Verification items for the finished model (mm, model axes). A direction names the side the tool comes from. Give positions to 0.01 mm unless a question says otherwise; leave off trailing zeros. Order: outer loops, then holes, each group sorted by start corner. A loop starts at its lowest first (then second) coordinate and runs counter-clockwise, first axis right, second up. Notation, with made-up numbers: (88, 51) -> (114, 51) arc R30 ccw to (114, 88) -> close; hole circle Ø3 at (76, 85). An arc over 180 degrees is marked (long way). One line per question, with ' | ' between items. Start each with the question number.
Q1. Section check B-B on y = -65. Record the cut outline in (x, z), plus the area to 3 significant figures.
Q2. Material ranges on probe 1 along X at (y, z) = (-66, 213.5); probe 2 along X at (y, z) = (-25.5, 204); probe 3 along Y at (x, z) = (89.5, 183), recorded low to high. Write a range as [from, to].
Q3. Mould release check, pull along Z, two halves, no side actions. Record for faces 1 (the flat face through (17, -127, 47)), 2 (the flat face through (159, -50, -71.583)), 3 (the cylindrical face through (24.996, -50.089, 186.226)): released by +Z, released by -Z, zero draft, split by the parting line, or undercut.
Q4. Section check C-C on x = 210.5. Record the cut outline in (y, z).
Q5. Section check A-A on z = 3. Record the cut outline in (x, y).
Q6. Go/stop test with a flat-tipped pin: pin 1 (2 mm diameter, centred on x = 72.5, z = 30.5, fed in from +Y). Record where the tip stops, or that it passes through.
Q7. Access from +Z, -Z, +X, -X, +Y, -Y to the whole of each face (thin tool, end or side, straight path). Record for faces 4 (the flat face through (230, -101.6, 85)), 5 (the flat face through (159, -50, 245.917)).
from build123d import *

# Parameters (mm, degrees)
F0_W        = 139.7
F0_H        = 317.5
F0_R        = 13.2493993782
F0_R_2      = 30.8467265461
F1_DEPTH    = 127
F2_T1_DEPTH = 266.7
F2_T3_DEPTH = 444.5
F3_DEPTH    = 288.29


# Not quite as in the source:
# - a fillet or chamfer that OpenCascade refuses, or shapes differently, is made with other operations: its cross-section is extruded or revolved along the edge and cut away or added


with BuildPart() as f1:
    # F0 (on Front) → F1 (new body)
    with BuildSketch(Plane.XZ):
        with Locations((18.042704469, 87.1669226885)):
            Rectangle(F0_W, F0_H)
        with Locations((-34.4466865063, 214.674949646)):
            Circle(F0_R, mode=Mode.SUBTRACT)
        with Locations((49.4750849903, 204.995855689)):
            Circle(F0_R_2, mode=Mode.SUBTRACT)
    extrude(amount=F1_DEPTH)

    # F2: fillet of radius 25.4 on 6 edges, made by hand

    # F2_s2 → F2_t1 (cut)
    with BuildSketch(Plane.YZ.offset(-115.307295531)):
        with BuildLine():
            ThreePointArc((-101.6, 245.9169226885), (-119.5605122421, 238.4774349306), (-127, 220.5169226885))
            Line((-127, 220.5169226885), (-127, 245.9169226885))
            Line((-127, 245.9169226885), (-101.6, 245.9169226885))
        make_face()
        with BuildLine():
            ThreePointArc((-101.6, -71.5830773115), (-119.5605122421, -64.1435895537), (-127, -46.1830773115))
            Line((-127, -46.1830773115), (-127, -71.5830773115))
            Line((-127, -71.5830773115), (-101.6, -71.5830773115))
        make_face()
    extrude(amount=F2_T1_DEPTH, mode=Mode.SUBTRACT)

    # F2_s4 → F2_t3 (cut)
    with BuildSketch(Plane.XY.offset(-135.0830773115)):
        with BuildLine():
            ThreePointArc((-51.807295531, -101.6), (-44.3678077732, -119.5605122421), (-26.407295531, -127))
            Line((-26.407295531, -127), (-51.807295531, -127))
            Line((-51.807295531, -127), (-51.807295531, -101.6))
        make_face()
        with BuildLine():
            ThreePointArc((87.892704469, -101.6), (80.4532167111, -119.5605122421), (62.492704469, -127))
            Line((62.492704469, -127), (87.892704469, -127))
            Line((87.892704469, -127), (87.892704469, -101.6))
        make_face()
    extrude(amount=F2_T3_DEPTH, mode=Mode.SUBTRACT)

    # F2_s5 → F2_t6 (revolve, cut)
    with BuildSketch(Plane.XY.offset(214.674949646)):
        with BuildLine():
            ThreePointArc((-21.197287128, -101.6), (-13.7577993702, -119.5605122421), (4.202712872, -127))
            Line((4.202712872, -127), (-21.197287128, -127))
            Line((-21.197287128, -127), (-21.197287128, -101.6))
        make_face()
    revolve(axis=Axis((-34.4466865063, -127, 214.674949646), (0, -1, 0)), mode=Mode.SUBTRACT)

    # F2_s7 → F2_t8 (revolve, cut)
    with BuildSketch(Plane.XY.offset(204.995855689)):
        with BuildLine():
            ThreePointArc((80.3218115364, -101.6), (87.7612992942, -119.5605122421), (105.7218115364, -127))
            Line((105.7218115364, -127), (80.3218115364, -127))
            Line((80.3218115364, -127), (80.3218115364, -101.6))
        make_face()
    revolve(axis=Axis((49.4750849903, -127, 204.995855689), (0, -1, 0)), mode=Mode.SUBTRACT)

    # F3 (add): a face of the model
    f3_faces = [f1.faces().sort_by_distance(p)[0] for p in [
        (87.892704469, -50.8, 87.1669226885),
    ]]
    extrude(f3_faces, amount=F3_DEPTH)


solid = f1.part
Filled in:
1) outline: (-51.81, -71.58) -> (376.18, -71.58) -> (376.18, 245.92) -> (-51.81, 245.92) -> close; hole circle Ø26.5 at (-34.45, 214.67); hole circle Ø61.69 at (49.48, 205) | area: 132,000 mm²
2) probe 1: [-51.81, -47.64], [-21.25, 19.82], [79.13, 376.18] | probe 2: [-51.81, -42.29], [-26.6, 18.64], [80.31, 376.18] | probe 3: [-101.6, 0]
3) face 1: zero draft | face 2: released by -Z | face 3: undercut
4) outline: (-101.6, -71.58) -> (0, -71.58) -> (0, 245.92) -> (-101.6, 245.92) -> close
5) outline: (-51.81, -101.6) arc R25.4 ccw to (-26.41, -127) -> (62.49, -127) arc R25.4 ccw to (87.89, -101.6) -> (376.18, -101.6) -> (376.18, 0) -> (-51.81, 0) -> close
6) pin 1: y = 0
7) face 4: +Z, -Z, +X, -Y | face 5: +Z, +X, -X, +Y, -Y
